Here's how the part is built. I have some questions about the finished solid (model axes, mm). Coordinates: 2 decimals unless noted, no trailing zeros.
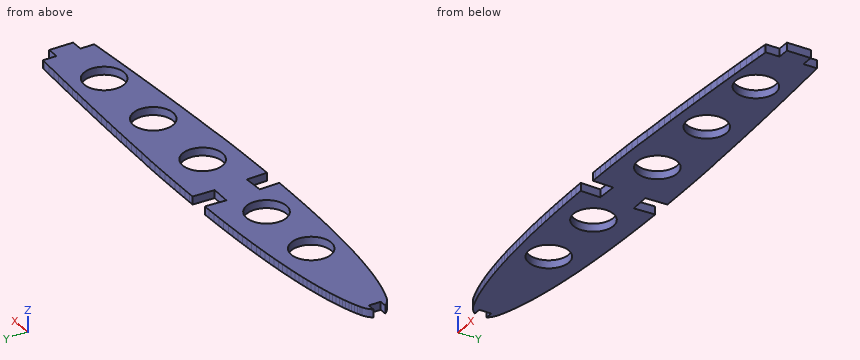
```python
from build123d import *

# Parameters (mm, degrees)
MODEL_R         = 4.999197418
EXTRUDE_1_DEPTH = 2


with BuildPart() as part:
    # Model → 凸台-拉伸1 (new body)
    with BuildSketch(Plane.XY):
        with BuildLine():
            Line((15.194094226, 17.721853744), (17.133079466, 17.721853744))
            Line((17.133079466, 17.721853744), (17.133079466, 14.721853744))
            Line((17.133079466, 14.721853744), (15.194094226, 14.721853744))
            ThreePointArc((15.194094226, 14.721853744), (16.131604287, 13.801473468), (17.226994751, 13.076115145))
            Line((17.226994751, 13.076115145), (17.74383436, 12.854853744))
            Line((17.74383436, 12.854853744), (18.36183436, 12.607853744))
            Line((18.36183436, 12.607853744), (19.09783436, 12.332853744))
            Line((19.09783436, 12.332853744), (19.84083436, 12.076853744))
            Line((19.84083436, 12.076853744), (20.58983436, 11.836853744))
            Line((20.58983436, 11.836853744), (21.45683436, 11.576853744))
            Line((21.45683436, 11.576853744), (22.32783436, 11.331853744))
            Line((22.32783436, 11.331853744), (23.20283436, 11.101853744))
            Line((23.20283436, 11.101853744), (24.19583436, 10.855853744))
            Line((24.19583436, 10.855853744), (25.19083436, 10.622853744))
            Line((25.19083436, 10.622853744), (26.18983436, 10.403853744))
            Line((26.18983436, 10.403853744), (27.30283436, 10.174853744))
            Line((27.30283436, 10.174853744), (28.41883436, 9.959853744))
            Line((28.41883436, 9.959853744), (29.53783436, 9.756853744))
            Line((29.53783436, 9.756853744), (30.76783436, 9.546853744))
            Line((30.76783436, 9.546853744), (31.99983436, 9.349853744))
            Line((31.99983436, 9.349853744), (33.23483436, 9.164853744))
            Line((33.23483436, 9.164853744), (34.57683436, 8.974853744))
            Line((34.57683436, 8.974853744), (35.91983436, 8.797853744))
            Line((35.91983436, 8.797853744), (37.26583436, 8.632853744))
            Line((37.26583436, 8.632853744), (38.71483436, 8.465853744))
            Line((38.71483436, 8.465853744), (40.16583436, 8.310853744))
            Line((40.16583436, 8.310853744), (41.61783436, 8.165853744))
            Line((41.61783436, 8.165853744), (43.16683436, 8.020853744))
            Line((43.16683436, 8.020853744), (44.71683436, 7.887853744))
            Line((44.71683436, 7.887853744), (46.26883436, 7.763853744))
            Line((46.26883436, 7.763853744), (47.91283436, 7.642853744))
            Line((47.91283436, 7.642853744), (49.55683436, 7.531853744))
            Line((49.55683436, 7.531853744), (51.20283436, 7.430853744))
            Line((51.20283436, 7.430853744), (52.93483436, 7.333853744))
            Line((52.93483436, 7.333853744), (54.66683436, 7.246853744))
            Line((54.66683436, 7.246853744), (56.40083436, 7.168853744))
            Line((56.40083436, 7.168853744), (58.21383436, 7.095853744))
            Line((58.21383436, 7.095853744), (60.02683436, 7.031853744))
            Line((60.02683436, 7.031853744), (61.84083436, 6.975853744))
            Line((61.84083436, 6.975853744), (63.72783436, 6.926853744))
            Line((63.72783436, 6.926853744), (65.61483436, 6.885853744))
            Line((65.61483436, 6.885853744), (67.50183436, 6.852853744))
            Line((67.50183436, 6.852853744), (69.45583436, 6.826853744))
            Line((69.45583436, 6.826853744), (71.40883436, 6.808853744))
            Line((71.40883436, 6.808853744), (71.24683436, 11.805853744))
            Line((71.24683436, 11.805853744), (76.24383436, 11.967853744))
            Line((76.24383436, 11.967853744), (76.40583436, 6.796082515))
            Line((76.40583436, 6.796082515), (77.38783436, 6.797853744))
            Line((77.38783436, 6.797853744), (79.40083436, 6.808853744))
            Line((79.40083436, 6.808853744), (81.46383436, 6.825853744))
            Line((81.46383436, 6.825853744), (83.52683436, 6.850853744))
            Line((83.52683436, 6.850853744), (85.58983436, 6.881853744))
            Line((85.58983436, 6.881853744), (87.69483436, 6.919853744))
            Line((87.69483436, 6.919853744), (89.79983436, 6.964853744))
            Line((89.79983436, 6.964853744), (91.90583436, 7.015853744))
            Line((91.90583436, 7.015853744), (94.04583436, 7.072853744))
            Line((94.04583436, 7.072853744), (97.601964333, 7.270653793))
            Line((97.601964333, 7.270653793), (97.90379269, 7.281104913))
            Line((97.90379269, 7.281104913), (100.06879269, 7.362104913))
            Line((100.06879269, 7.362104913), (102.23479269, 7.447104913))
            Line((102.23479269, 7.447104913), (104.41879269, 7.538104913))
            Line((104.41879269, 7.538104913), (106.60179269, 7.634104913))
            Line((106.60179269, 7.634104913), (108.78479269, 7.734104913))
            Line((108.78479269, 7.734104913), (110.97679269, 7.840104913))
            Line((110.97679269, 7.840104913), (113.16779269, 7.951104913))
            Line((113.16779269, 7.951104913), (115.35879269, 8.067104913))
            Line((115.35879269, 8.067104913), (117.55079269, 8.189104913))
            Line((117.55079269, 8.189104913), (119.74079269, 8.314104913))
            Line((119.74079269, 8.314104913), (121.93279269, 8.442104913))
            Line((121.93279269, 8.442104913), (124.11679269, 8.572104913))
            Line((124.11679269, 8.572104913), (126.29979269, 8.704104913))
            Line((126.29979269, 8.704104913), (128.48279269, 8.840104913))
            Line((128.48279269, 8.840104913), (130.64879269, 8.980104913))
            Line((130.64879269, 8.980104913), (132.81379269, 9.124104913))
            Line((132.81379269, 9.124104913), (134.97979269, 9.271104913))
            Line((134.97979269, 9.271104913), (137.11979269, 9.419104913))
            Line((137.11979269, 9.419104913), (139.25979269, 9.570104913))
            Line((139.25979269, 9.570104913), (141.39979269, 9.724104913))
            Line((141.39979269, 9.724104913), (142.088794604, 9.774487769))
            Line((142.088794604, 9.774487769), (142.086848241, 13.259514384))
            Line((142.086848241, 13.259514384), (145.086848241, 13.259514384))
            Line((145.086848241, 13.259514384), (145.086848241, 19.259514384))
            Line((145.086848241, 19.259514384), (142.086848241, 19.259514384))
            Line((142.086848241, 19.259514384), (142.086848241, 22.673864384))
            Line((142.086848241, 22.673864384), (141.39979269, 22.724104913))
            Line((141.39979269, 22.724104913), (139.25979269, 22.878104913))
            Line((139.25979269, 22.878104913), (137.11979269, 23.029104913))
            Line((137.11979269, 23.029104913), (134.97979269, 23.177104913))
            Line((134.97979269, 23.177104913), (132.81379269, 23.324104913))
            Line((132.81379269, 23.324104913), (130.64879269, 23.468104913))
            Line((130.64879269, 23.468104913), (128.48279269, 23.608104913))
            Line((128.48279269, 23.608104913), (126.29979269, 23.744104913))
            Line((126.29979269, 23.744104913), (124.11679269, 23.877104913))
            Line((124.11679269, 23.877104913), (121.93279269, 24.006104913))
            Line((121.93279269, 24.006104913), (119.74079269, 24.134104913))
            Line((119.74079269, 24.134104913), (117.55079269, 24.260104913))
            Line((117.55079269, 24.260104913), (115.35879269, 24.381104913))
            Line((115.35879269, 24.381104913), (113.16779269, 24.497104913))
            Line((113.16779269, 24.497104913), (110.97679269, 24.608104913))
            Line((110.97679269, 24.608104913), (108.78479269, 24.714104913))
            Line((108.78479269, 24.714104913), (106.60179269, 24.814104913))
            Line((106.60179269, 24.814104913), (104.41879269, 24.910104913))
            Line((104.41879269, 24.910104913), (102.23479269, 25.001104913))
            Line((102.23479269, 25.001104913), (100.06879269, 25.086104913))
            Line((100.06879269, 25.086104913), (97.90379269, 25.167104913))
            Line((97.90379269, 25.167104913), (97.601514741, 25.177571601))
            Line((97.601514741, 25.177571601), (94.04583436, 25.370853744))
            Line((94.04583436, 25.370853744), (91.90583436, 25.427853744))
            Line((91.90583436, 25.427853744), (89.79983436, 25.478853744))
            Line((89.79983436, 25.478853744), (87.69483436, 25.523853744))
            Line((87.69483436, 25.523853744), (85.58983436, 25.561853744))
            Line((85.58983436, 25.561853744), (83.52683436, 25.592853744))
            Line((83.52683436, 25.592853744), (81.46383436, 25.617853744))
            Line((81.46383436, 25.617853744), (79.40083436, 25.635853744))
            Line((79.40083436, 25.635853744), (77.38783436, 25.645853744))
            Line((77.38783436, 25.645853744), (76.190756889, 25.64823362))
            Line((76.190756889, 25.64823362), (76.02683436, 20.178853744))
            Line((76.02683436, 20.178853744), (71.02883436, 20.340853744))
            Line((71.02883436, 20.340853744), (71.243114412, 25.633326371))
            Line((71.243114412, 25.633326371), (69.45583436, 25.616853744))
            Line((69.45583436, 25.616853744), (67.50183436, 25.591853744))
            Line((67.50183436, 25.591853744), (65.61483436, 25.558853744))
            Line((65.61483436, 25.558853744), (63.72783436, 25.516853744))
            Line((63.72783436, 25.516853744), (61.84083436, 25.467853744))
            Line((61.84083436, 25.467853744), (60.02683436, 25.411853744))
            Line((60.02683436, 25.411853744), (58.21383436, 25.347853744))
            Line((58.21383436, 25.347853744), (56.40083436, 25.274853744))
            Line((56.40083436, 25.274853744), (54.66683436, 25.196853744))
            Line((54.66683436, 25.196853744), (52.93483436, 25.109853744))
            Line((52.93483436, 25.109853744), (51.20283436, 25.013853744))
            Line((51.20283436, 25.013853744), (49.55683436, 24.911853744))
            Line((49.55683436, 24.911853744), (47.91283436, 24.801853744))
            Line((47.91283436, 24.801853744), (46.26883436, 24.680853744))
            Line((46.26883436, 24.680853744), (44.71683436, 24.556853744))
            Line((44.71683436, 24.556853744), (43.16683436, 24.422853744))
            Line((43.16683436, 24.422853744), (41.61783436, 24.277853744))
            Line((41.61783436, 24.277853744), (40.16583436, 24.132853744))
            Line((40.16583436, 24.132853744), (38.71483436, 23.977853744))
            Line((38.71483436, 23.977853744), (37.26583436, 23.810853744))
            Line((37.26583436, 23.810853744), (35.91983436, 23.645853744))
            Line((35.91983436, 23.645853744), (34.57683436, 23.468853744))
            Line((34.57683436, 23.468853744), (33.23483436, 23.279853744))
            Line((33.23483436, 23.279853744), (31.99983436, 23.093853744))
            Line((31.99983436, 23.093853744), (30.76783436, 22.896853744))
            Line((30.76783436, 22.896853744), (29.53783436, 22.686853744))
            Line((29.53783436, 22.686853744), (28.41883436, 22.483853744))
            Line((28.41883436, 22.483853744), (27.30283436, 22.268853744))
            Line((27.30283436, 22.268853744), (26.18983436, 22.039853744))
            Line((26.18983436, 22.039853744), (25.19083436, 21.820853744))
            Line((25.19083436, 21.820853744), (24.19583436, 21.588853744))
            Line((24.19583436, 21.588853744), (23.20283436, 21.341853744))
            Line((23.20283436, 21.341853744), (22.32783436, 21.111853744))
            Line((22.32783436, 21.111853744), (21.45683436, 20.867853744))
            Line((21.45683436, 20.867853744), (20.58983436, 20.606853744))
            Line((20.58983436, 20.606853744), (19.84083436, 20.366853744))
            Line((19.84083436, 20.366853744), (19.09783436, 20.110853744))
            Line((19.09783436, 20.110853744), (18.36183436, 19.836853744))
            Line((18.36183436, 19.836853744), (17.74383436, 19.588853744))
            Line((17.74383436, 19.588853744), (17.222488144, 19.365660445))
            ThreePointArc((17.222488144, 19.365660445), (16.089203867, 18.690706241), (15.194094226, 17.721853744))
        make_face()
        with Locations((62.354774691, 15.571631352)):
            Circle(MODEL_R, mode=Mode.SUBTRACT)
        with Locations((88.444584336, 15.571631352)):
            Circle(MODEL_R, mode=Mode.SUBTRACT)
        with Locations((108.610323656, 15.571631352)):
            Circle(MODEL_R, mode=Mode.SUBTRACT)
        with Locations((128.651429135, 15.571631352)):
            Circle(MODEL_R, mode=Mode.SUBTRACT)
        with Locations((44.129846481, 15.571631352)):
            Circle(MODEL_R, mode=Mode.SUBTRACT)
    extrude(amount=EXTRUDE_1_DEPTH)


solid = part.part
```
1) Will these pins go through, and if not, where does the flat tip stop? pin 1 (1.5 mm diameter, centred on x = 111.5, y = 16, fed in from +Z); pin 2 (0.6 mm diameter, centred on x = 16, z = 0.5, fed in from -Y); pin 3 (1 mm diameter, centred on y = 16, z = 0.5, fed in from -X); pin 4 (0.6 mm diameter, centred on y = 20.5, z = 1, fed in from +X).
Values follow:
pin 1: passes through
pin 2: stops at y = 13.67
pin 3: stops at x = 17.13
pin 4: stops at x = 142.09
2) I need wall thicknesses on probe 1 along X at (y, z) = (15.25, 1); probe 2 along X at (y, z) = (19, 1.35); probe 3 along Y at (x, z) = (86.5, 1.2). Which ranges of each line are inside material? Lowest first, please.
Values follow:
probe 1: x = 17.13 to 39.14, 49.12 to 57.37, 67.34 to 83.46, 93.43 to 103.62, 113.6 to 123.66, 133.64 to 145.09
probe 2: x = 16.52 to 40.49, 47.77 to 58.72, 65.99 to 84.81, 92.08 to 104.97, 112.25 to 125.01, 132.29 to 145.09
probe 3: y = 6.9 to 10.97, 20.18 to 25.55
3) Imagine slicing it at A-A on z = 1. Count the separate pieces of the cut face and the enclosed holes in it, then the cut area to 3 significant figures.
Values follow:
separate pieces: 1
enclosed holes: 5
area: 1,600 mm2
